from build123d import *

# Parameters (mm, degrees)
SKETCH1_W           = 100
SKETCH1_H           = 75
BOSS_EXTRUDE1_DEPTH = 9
SKETCH2_W           = 40
SKETCH2_H           = 31.155322697
BOSS_EXTRUDE2_DEPTH = 9
FILLET1_R           = 10
FILLET2_R           = 15
SKETCH3_R           = 7.5
CUT_EXTRUDE1_DEPTH  = 127.289350303
SKETCH4_W           = 25
SKETCH4_H           = 15
CUT_EXTRUDE2_DEPTH  = 3
FILLET3_R           = 5
SKETCH5_R           = 1.5
SKETCH5_R_2         = 2.5
CUT_EXTRUDE3_DEPTH  = 7
SKETCH6_R           = 7.5
BOSS_EXTRUDE3_DEPTH = 7


with BuildPart() as part:
    # Sketch1 → Boss-Extrude1 (new body)
    with BuildSketch(Plane(origin=(0, 0, 0), x_dir=(1, 0, 0), z_dir=(0, 1, 0))):
        with Locations((50, -37.5)):
            Rectangle(SKETCH1_W, SKETCH1_H)
    extrude(amount=BOSS_EXTRUDE1_DEPTH)

    # Sketch2 → Boss-Extrude2 (add)
    with BuildSketch(Plane(origin=(0, 9, 0), x_dir=(1, 0, 0), z_dir=(0, 1, 0))):
        with Locations((30, -36.922338651)):
            Rectangle(SKETCH2_W, SKETCH2_H)
    extrude(amount=BOSS_EXTRUDE2_DEPTH)

    # Fillet1
    fillet1_edges = [part.edges().sort_by_distance(p)[0] for p in [
        (10, 13.5, 21.344677303),
        (10, 13.5, 52.5),
    ]]
    fillet(fillet1_edges, radius=FILLET1_R)

    # Fillet2
    fillet2_edges = [part.edges().sort_by_distance(p)[0] for p in [
        (50, 13.5, 52.5),
        (50, 13.5, 21.344677303),
    ]]
    fillet(fillet2_edges, radius=FILLET2_R)

    # Sketch3 → Cut-Extrude1 (cut, through all)
    with BuildSketch(Plane(origin=(0, 18, 0), x_dir=(1, 0, 0), z_dir=(0, 1, 0))):
        with Locations(Location((30, -36.922338651, 0), (0, 0, 270))):
            Circle(SKETCH3_R)
    extrude(amount=-CUT_EXTRUDE1_DEPTH, mode=Mode.SUBTRACT)

    # Sketch4 → Cut-Extrude2 (cut)
    with BuildSketch(Plane(origin=(0, 9, 0), x_dir=(1, 0, 0), z_dir=(0, 1, 0))):
        with Locations((67.5, -60)):
            Rectangle(SKETCH4_W, SKETCH4_H)
        with Locations((67.5, -15)):
            Rectangle(SKETCH4_W, SKETCH4_H)
    extrude(amount=-CUT_EXTRUDE2_DEPTH, mode=Mode.SUBTRACT)

    # Fillet3
    fillet3_edges = [part.edges().sort_by_distance(p)[0] for p in [
        (55, 7.5, 67.5),
        (55, 7.5, 52.5),
        (80, 7.5, 52.5),
        (80, 7.5, 67.5),
        (80, 7.5, 22.5),
        (55, 7.5, 22.5),
        (55, 7.5, 7.5),
        (80, 7.5, 7.5),
    ]]
    fillet(fillet3_edges, radius=FILLET3_R)

    # Sketch5 → Cut-Extrude3 (cut)
    with BuildSketch(Plane(origin=(0, 6, 0), x_dir=(1, 0, 0), z_dir=(0, 1, 0))):
        with Locations(Location((62.5, -60, 0), (0, 0, 270))):
            Circle(SKETCH5_R)
        with Locations(Location((72.5, -60, 0), (0, 0, 270))):
            Circle(SKETCH5_R_2)
        with Locations(Location((72.5, -15, 0), (0, 0, 270))):
            Circle(SKETCH5_R_2)
        with Locations(Location((62.5, -15, 0), (0, 0, 270))):
            Circle(SKETCH5_R)
    extrude(amount=-CUT_EXTRUDE3_DEPTH, mode=Mode.SUBTRACT)

    # Sketch6 → Boss-Extrude3 (add)
    with BuildSketch(Plane(origin=(0, 9, 0), x_dir=(1, 0, 0), z_dir=(0, 1, 0))):
        with Locations(Location((80, -37.5, 0), (0, 0, 270))):
            Circle(SKETCH6_R)
    extrude(amount=BOSS_EXTRUDE3_DEPTH)

    # Sketch7 → Revolve1 (revolve)
    with BuildSketch(Plane(origin=(0, 16, 0), x_dir=(1, 0, 0), z_dir=(0, 1, 0))):
        with BuildLine():
            Line((74, -37.5), (86, -37.5))
            ThreePointArc((86, -37.5), (80, -43.5), (74, -37.5))
        make_face()
    revolve(axis=Axis((72.5, 16, 37.5), (1, 0, 0)))


solid = part.part
Verification items for the finished model (mm, model axes). A direction names the side the tool comes from. Round coordinates to 2 decimals unless told otherwise and drop trailing zeros. Loops run counter-clockwise (first coordinate to the right, second up) from the corner with the lowest first, then second, coordinate; pieces in that order, holes last. Notation, with made-up numbers: (75.25, 30) - (102.25, 30) arc R25 cw to (102.25, 60) - close; hole circle Ø5 at (61, 2). An arc over 180 degrees is marked (long way). Use a Markdown table: item, result. Add a question column.
1. Section check D-D, the plane y = 2.5. Record the boundary of the cut face in (x, z), plus the area to 3 significant figures.
2. Section check B-B, the plane z = 60. Record the boundary of the cut face in (x, y), plus the area to 3 significant figures.
3. Section check A-A, the plane y = 11.5. Record the boundary of the cut face in (x, z), plus the area to 3 significant figures.
4. Gauge pin test, flat ends, axial feed: pin 1 (4.5 mm diameter, centred on x = 65.5, z = 16.5, fed in from +Y); pin 2 (1.5 mm diameter, centred on y = 12, z = 38.5, fed in from +X); pin 3 (2 mm diameter, centred on y = 18, z = 35, fed in from +X). Record the tip position at first contact, or that the pin passes through.
5. Release check for a two-part mould opening along X. For faces 4 (the face through (49, 0, 37)), 5 (the face through (100, 4, 38)), 6 (the face through (67, 6, 60)) record: released by +X, released by -X, zero draft, split by the parting line, or undercut.
6. Access from +Z, -Z, +X, -X, +Y, -Y to the whole of each face (thin tool, end or side, straight path). Record for faces 1 (the face through (67, 8, 7.5)), 2 (the face through (27, 13, 52.5)), 3 (the face through (62.95, 3.04, 61.43)).
7. Section check C-C, the plane x = 62.5. Record the boundary of the cut face in (y, z).
8. Thickness scan on probe 1 along X at (y, z) = (3.1, 15); probe 2 along X at (y, z) = (8.5, 57.5); probe 3 along X at (y, z) = (15.75, 34.5). Record the ranges inside material, lowest first. Write a range as [from, to].
Checks:
| question | item | result |
|---|---|---|
| 1 | outline | (0, 0) - (100, 0) - (100, 75) - (0, 75) - close; hole circle Ø15 at (30, 36.92); hole circle Ø3 at (62.5, 15); hole circle Ø3 at (62.5, 60); hole circle Ø5 at (72.5, 15); hole circle Ø5 at (72.5, 60) |
| 1 | area | 7,270 mm^2 |
| 2 | outline | (0, 0) - (61, 0) - (61, 6) - (55, 6) - (55, 9) - (0, 9) - close; (64, 0) - (70, 0) - (70, 6) - (64, 6) - close; (75, 0) - (100, 0) - (100, 9) - (80, 9) - (80, 6) - (75, 6) - close |
| 2 | area | 777 mm^2 |
| 3 | outline | (10, 31.34) arc R10 ccw to (20, 21.34) - (35, 21.34) arc R15 ccw to (50, 36.34) - (50, 37.5) arc R15 ccw to (35, 52.5) - (20, 52.5) arc R10 ccw to (10, 42.5) - close; circle Ø15 at (80, 37.5); hole circle Ø15 at (30, 36.92) |
| 3 | area | 1,110 mm^2 |
| 4 | pin 1 | stops at y = 6 |
| 4 | pin 2 | stops at x = 87.5 |
| 4 | pin 3 | stops at x = 85.58 |
| 5 | face 4 | zero draft |
| 5 | face 5 | released by +X |
| 5 | face 6 | undercut |
| 6 | face 1 | +Y |
| 6 | face 2 | +Z, +X, -X, +Y |
| 6 | face 3 | +Y, -Y |
| 7 | outline | (0, 0) - (9, 0) - (9, 7.5) - (6, 7.5) - (6, 13.5) - (0, 13.5) - close; (0, 16.5) - (6, 16.5) - (6, 22.5) - (9, 22.5) - (9, 52.5) - (6, 52.5) - (6, 58.5) - (0, 58.5) - close; (0, 61.5) - (6, 61.5) - (6, 67.5) - (9, 67.5) - (9, 75) - (0, 75) - close |
| 8 | probe 1 | x = [0, 61], [64, 70], [75, 100] |
| 8 | probe 2 | x = [0, 55], [80, 100] |
| 8 | probe 3 | x = [10, 22.9], [37.1, 49.89], [73.13, 86.87] |
